Work out the finished part from the listing and answer in its coordinate system (mm). Face numbers are marked on the shaded views. A direction names the side the tool comes from. Round coordinates to 2 decimals unless told otherwise and drop trailing zeros. Order: outer loops, then holes, each group sorted by start corner. A loop starts at its lowest first (then second) coordinate and runs counter-clockwise, first axis right, second up. Notation, with made-up numbers: M 10,43.5 L 49,43.5 A22 ccw 49,79.5 Z; hole C -31,-33 d4. An arc over 180 degrees is marked long. Return JSON: item names as keys, results as strings.
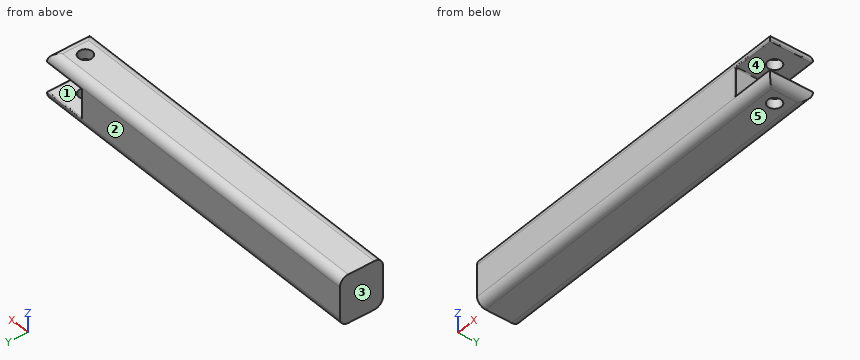
from build123d import *

# Parameters (mm, degrees)
SKETCH1_W               = 212.2
SKETCH1_H               = 25.4
BOSS_EXTRUDE1_DEPTH     = 14.2875
CUT_EXTRUDE2_DEPTH      = 108.808314412
CUT_EXTRUDE2_DEPTH_BACK = 108.808314412
SKETCH2_R               = 4
CUT_EXTRUDE3_DEPTH      = 108.808314412
CUT_EXTRUDE3_DEPTH_BACK = 108.808314412
SKETCH3_W               = 25
SKETCH3_H               = 17
FILLET3_R               = 5
FILLET4_R               = 0.5


with BuildPart() as part:
    # Sketch1 → Boss-Extrude1 (new, symmetric)
    with BuildSketch(Plane.XY):
        Rectangle(SKETCH1_W, SKETCH1_H)
    extrude(amount=BOSS_EXTRUDE1_DEPTH, both=True)

    # Sketch2 → Cut-Extrude2 (cut, two sides: drawn at the far end of the back side and taken through both)
    with BuildSketch(Plane.XY.offset(-CUT_EXTRUDE2_DEPTH_BACK)):
        with Locations((93.9, 0)):
            Circle(SKETCH2_R)
    extrude(amount=CUT_EXTRUDE2_DEPTH + CUT_EXTRUDE2_DEPTH_BACK, mode=Mode.SUBTRACT)

    # Sketch3 → Cut-Extrude3 (cut, two sides: drawn at the far end of the back side and taken through both)
    with BuildSketch(Plane(origin=(0, 0, 0), x_dir=(1, 0, 0), z_dir=(0, 1, 0)).offset(-CUT_EXTRUDE3_DEPTH_BACK)):
        with Locations((93.6, 0)):
            Rectangle(SKETCH3_W, SKETCH3_H)
    extrude(amount=CUT_EXTRUDE3_DEPTH + CUT_EXTRUDE3_DEPTH_BACK, mode=Mode.SUBTRACT)

    # Fillet3
    fillet3_edges = [part.edges().sort_by_distance(p)[0] for p in [
        (106.1, 0, 14.2875),
        (0, 12.7, 14.2875),
        (0, 12.7, -14.2875),
        (106.1, 0, -14.2875),
        (0, -12.7, -14.2875),
        (0, -12.7, 14.2875),
    ]]
    fillet(fillet3_edges, radius=FILLET3_R)

    # Fillet4
    fillet4_edges = [part.edges().sort_by_distance(p)[0] for p in [
        (106.1, 0, 8.5),
        (93.6, -12.7, 8.5),
        (81.1, 0, -8.5),
        (93.6, -12.7, -8.5),
        (106.1, 0, -8.5),
        (81.1, 0, 8.5),
        (81.1, -12.7, 0),
        (93.6, 12.7, -8.5),
        (81.1, 12.7, 0),
        (93.6, 12.7, 8.5),
    ]]
    fillet(fillet4_edges, radius=FILLET4_R)


solid = part.part
Item 1: The mould has two halves that part along Z. Classify the marked faces 3, 4 and 5: pulls with the +Z half, pulls with the -Z half, needs draft (parallel to the pull), parting line crosses it, or undercut.
Output:
{"face 3": "needs draft", "face 4": "undercut", "face 5": "pulls with the -Z half"}
Item 2: Find section D-D (z = -11.25). Determine the outline of the cut face in (x, y).
Output:
{"outline": "M -106.1,-12.3 L 105.7,-12.3 L 105.7,12.3 L -106.1,12.3 Z; hole C 93.9,0 d8"}
Item 3: Find section C-C (x = 70.5). Determine the outline of the cut face in (y, z).
Output:
{"outline": "M -12.7,-9.29 A5 ccw -7.7,-14.29 L 7.7,-14.29 A5 ccw 12.7,-9.29 L 12.7,9.29 A5 ccw 7.7,14.29 L -7.7,14.29 A5 ccw -12.7,9.29 Z"}
Item 4: Find section B-B (y = 0). Determine the outline of the cut face in (x, z).
Output:
{"outline": "M -106.1,-14.29 L 89.9,-14.29 L 89.9,-8.5 L 81.6,-8.5 A0.5 cw 81.1,-8 L 81.1,8 A0.5 cw 81.6,8.5 L 89.9,8.5 L 89.9,14.29 L -106.1,14.29 Z; M 97.9,-14.29 L 101.1,-14.29 A5 ccw 106.1,-9.29 L 106.1,-9 A0.5 ccw 105.6,-8.5 L 97.9,-8.5 Z; M 97.9,8.5 L 105.6,8.5 A0.5 ccw 106.1,9 L 106.1,9.29 A5 ccw 101.1,14.29 L 97.9,14.29 Z"}
Item 5: Which of the six approach directions +Z, -Z, +X, -X, +Y, -Y give full straight-line access (tool end or side, diameter ignored) to the marked faces 1 and 2?
Output:
{"face 1": "+X, +Y, -Y", "face 2": "+Z, -Z, +X, -X, +Y"}
Item 6: Each of these flat-tipped pins is pushed along its axis until it touches: pin 1 (6.5 mm diameter, centred on x = 93.9, y = 0, fed in from -Z); pin 2 (2 mm diameter, centred on x = 15, z = -10.5, fed in from +Y). Where does it stop, or does it pass through?
Output:
{"pin 1": "passes through", "pin 2": "stops at y = 12.7"}
Item 7: Find section A-A (x = 93.9). Determine the outline of the cut face in (y, z).
Output:
{"outline": "M -12.7,-9.29 A5 ccw -7.7,-14.29 L -4,-14.29 L -4,-8.5 L -12.2,-8.5 A0.5 ccw -12.7,-9 Z; M -12.7,9 A0.5 ccw -12.2,8.5 L -4,8.5 L -4,14.29 L -7.7,14.29 A5 ccw -12.7,9.29 Z; M 4,-14.29 L 7.7,-14.29 A5 ccw 12.7,-9.29 L 12.7,-9 A0.5 ccw 12.2,-8.5 L 4,-8.5 Z; M 4,8.5 L 12.2,8.5 A0.5 ccw 12.7,9 L 12.7,9.29 A5 ccw 7.7,14.29 L 4,14.29 Z"}
Item 8: Consider line 1 along Y through (x, z) = (93.9, -9.8); line 2 along Y through (x, z) = (93.9, -11.5); line 3 along X through (y, z) = (-7.5, 0.75). Determine where each line is inside the solid, lowest interval first. Write a range as [from, to].
Output:
{"line 1": "y = [-12.67, -4], [4, 12.67]", "line 2": "y = [-12.18, -4], [4, 12.18]", "line 3": "x = [-106.1, 81.1]"}
